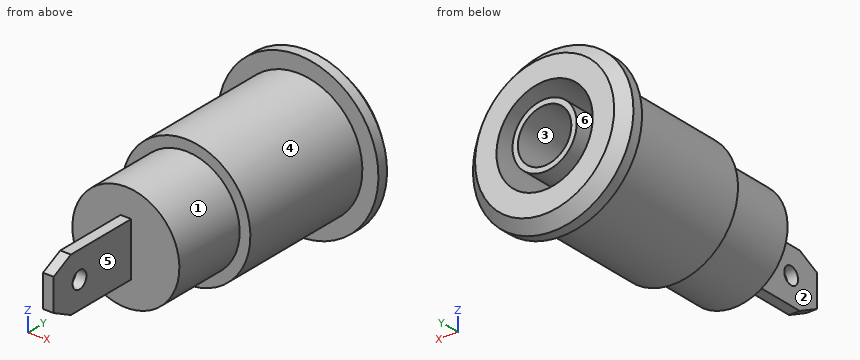
```python
from build123d import *

# Parameters (mm, degrees)
CHANFREIN1_SIZE         = 1
ESQUISSE2_R             = 4.5
ENL_V_MAT_EXTRU_1_DEPTH = 12
ESQUISSE3_R             = 3
BOSS_EXTRU_1_DEPTH      = 12
ESQUISSE4_R             = 2.5
ENL_V_MAT_EXTRU_2_DEPTH = 12
ESQUISSE5_W             = 5
ESQUISSE5_H             = 9
BOSS_EXTRU_2_DEPTH      = 1
ENL_V_MAT_EXTRU_3_DEPTH = 1
ENL_V_MAT_EXTRU_4_DEPTH = 1
ESQUISSE8_R             = 0.8
ENL_V_MAT_EXTRU_5_DEPTH = 1


with BuildPart() as part:
    # Esquisse1 → Base-Révolution (revolve)
    with BuildSketch(Plane(origin=(0, 0, 0), x_dir=(0, 0, -1), z_dir=(1, 0, 0)), mode=Mode.PRIVATE) as base_r_volution_sk:
        Polygon((0, 0), (7.5, 0), (7.5, -2), (6, -2), (6, -15), (5, -15), (5, -22), (0, -22), align=None)
    revolve(base_r_volution_sk.sketch.rotate(Axis((0, 10, 0), (0, -1, 0)), 180), axis=Axis((0, 10, 0), (0, -1, 0)))

    # Chanfrein1
    chanfrein1_edges = [part.edges().sort_by_distance(p)[0] for p in [
        (0, 0, -7.5),
    ]]
    chamfer(chanfrein1_edges, length=CHANFREIN1_SIZE)

    # Esquisse2 → Enlèv. mat.-Extru.1 (cut)
    with BuildSketch(Plane(origin=(0, 0, 0), x_dir=(-1, 0, 0), z_dir=(0, 1, 0))):
        with Locations(Location((0, 0, 0), (0, 0, 90))):
            Circle(ESQUISSE2_R)
    extrude(amount=-ENL_V_MAT_EXTRU_1_DEPTH, mode=Mode.SUBTRACT)

    # Esquisse3 → Boss.-Extru.1 (add)
    with BuildSketch(Plane(origin=(0, -12, 0), x_dir=(-1, 0, 0), z_dir=(0, 1, 0))):
        with Locations(Location((0, 0, 0), (0, 0, 90))):
            Circle(ESQUISSE3_R)
    extrude(amount=BOSS_EXTRU_1_DEPTH)

    # Esquisse4 → Enlèv. mat.-Extru.2 (cut)
    with BuildSketch(Plane(origin=(0, 0, 0), x_dir=(-1, 0, 0), z_dir=(0, 1, 0))):
        with Locations(Location((0, 0, 0), (0, 0, 90))):
            Circle(ESQUISSE4_R)
    extrude(amount=-ENL_V_MAT_EXTRU_2_DEPTH, mode=Mode.SUBTRACT)

    # Esquisse5 → Boss.-Extru.2 (add)
    with BuildSketch(Plane(origin=(0.5, 0, 0), x_dir=(0, 0, -1), z_dir=(1, 0, 0))):
        with Locations((0, -26.5)):
            Rectangle(ESQUISSE5_W, ESQUISSE5_H)
    extrude(amount=-BOSS_EXTRU_2_DEPTH)

    # Esquisse6 → Enlèv. mat.-Extru.3 (cut)
    with BuildSketch(Plane(origin=(0.5, 0, 0), x_dir=(0, 0, -1), z_dir=(1, 0, 0))):
        Polygon((-2.5, -29), (-1.5, -31), (-2.5, -31), align=None)
    extrude(amount=-ENL_V_MAT_EXTRU_3_DEPTH, mode=Mode.SUBTRACT)

    # Esquisse7 → Enlèv. mat.-Extru.4 (cut)
    with BuildSketch(Plane(origin=(0.5, 0, 0), x_dir=(0, 0, -1), z_dir=(1, 0, 0))):
        Polygon((2.5, -31), (2.5, -29), (1.5, -31), align=None)
    extrude(amount=-ENL_V_MAT_EXTRU_4_DEPTH, mode=Mode.SUBTRACT)

    # Esquisse8 → Enlèv. mat.-Extru.5 (cut)
    with BuildSketch(Plane(origin=(0.5, 0, 0), x_dir=(0, 0, -1), z_dir=(1, 0, 0))):
        with Locations((0, -28)):
            Circle(ESQUISSE8_R)
    extrude(amount=-ENL_V_MAT_EXTRU_5_DEPTH, mode=Mode.SUBTRACT)


solid = part.part
```
The model under review builds one solid part; all positions refer to its coordinate system, in mm. Face numbers are marked on the shaded views. A direction names the side the tool comes from. Round coordinates to 2 decimals unless told otherwise and drop trailing zeros. Loops run counter-clockwise (first coordinate to the right, second up) from the corner with the lowest first, then second, coordinate; pieces in that order, holes last. Notation, with made-up numbers: (-12, 8) -> (-4, 8) arc R14 cw to (-4, 23) -> close; hole circle Ø8 at (85, 64). An arc over 180 degrees is marked (long way). Answer as a JSON object with one key per item and string values. Group by question number.
1) We need section D-D on y = -3. Write out the cut boundary in (x, z), then the cut area to 3 significant figures.
2) For the marked faces 4, 5 and 6, list the 3-axis set-ups (+Z, -Z, +X, -X, +Y, -Y) from which the entire face can be reached by the end or side of a thin tool; tool diameter is ignored.
3) We need section B-B on y = -28. Write out the cut boundary in (x, z), then the cut area to 3 significant figures.
4) For line 1 (X direction, y = -3.5, z = 0); line 2 (Y direction, x = 0.2, z = 0); line 3 (X direction, y = -4, z = 2.75), list the stretches that pass through material, from the lowest coordinate up. Write a range as [from, to].
5) Mouldability with a two-part tool opening along Z and no side actions: class the marked faces 1, 2 and 3 as released by +Z, released by -Z, zero draft, split by the parting line, or undercut.
6) For pin 1 Ø8 at (x, y) = (6, -21) entering from -Z; pin 2 Ø1.5 at (x, y) = (-5, -17.5) entering from -Z; pin 3 Ø2.5 at (y, z) = (-28.5, 0.5) entering from -X; pin 4 Ø8 at (x, z) = (-2.5, 2.5) entering from +Y, all flat-tipped, find the tip position at first contact; note any pin that passes through.
Result set:
{
 "1": {"outline": "circle Ø12 at (0, 0); circle Ø6 at (0, 0); hole circle Ø9 at (0, 0); hole circle Ø5 at (0, 0)", "area": "58.1 mm²"},
 "2": {"face 4": "-Y", "face 5": "+Z, -Z, +X, -Y", "face 6": "+Y"},
 "3": {"outline": "(-0.5, -2.5) -> (0.5, -2.5) -> (0.5, -0.8) -> (-0.5, -0.8) -> close; (-0.5, 0.8) -> (0.5, 0.8) -> (0.5, 2.5) -> (-0.5, 2.5) -> close", "area": "3.40 mm²"},
 "4": {"line 1": "[-6, -4.5], [-3, -2.5], [2.5, 3], [4.5, 6]", "line 2": "[-31, -28.8], [-27.2, -12]", "line 3": "[-5.33, -3.56], [-1.2, 1.2], [3.56, 5.33]"},
 "5": {"face 1": "split by the parting line", "face 2": "zero draft", "face 3": "undercut"},
 "6": {"pin 1": "z = -4.58", "pin 2": "z = -2.63", "pin 3": "x = -0.5", "pin 4": "y = 0"}
}
